Input: dimensioned drawing with shaded views. Units: mm. Origin: part minimum x, y, z. A direction names the side the tool comes from. Give positions to 0.01 mm unless a question says otherwise; leave off trailing zeros. Loops run counter-clockwise (first coordinate to the right, second up) from the corner with the lowest first, then second, coordinate; pieces in that order, holes last. Notation, with made-up numbers: M 26.25,-7.5 L 73.25,-7.5 A15 cw 73.25,17.5 Z; hole C 24,51.5 d11. An arc over 180 degrees is marked long. Use CSV: the item, a comma, the result in double quotes. Start each with the question number.
Q1. Section A-A, the plane z = 10. Output: boundary loops of the cut face in (x, y).
Q2. Reachability of the marked faces 4 and 5 from +Z, -Z, +X, -X, +Y, -Y: full face, straight path, thin tool, end or side. Return the list, or none.
Q3. Section B-B, the plane y = 1.65. Output: boundary loops of the cut face in (x, z).
Q4. Pin query (flat end, axial travel): pin 1 (2.5 mm diameter, centred on x = 10, z = 2.5, fed in from +Y); pin 2 (3 mm diameter, centred on x = 17, z = 15, fed in from +Y); pin 3 (1.5 mm diameter, centred on x = 6, y = 1, fed in from -Z); pin 4 (1 mm diameter, centred on y = 2, z = 5, fed in from +X). Return the tip coordinate at first contact, or that it passes through.
Q5. Section D-D, the plane z = 3.5. Output: boundary loops of the cut face in (x, y), plus the area to 3 significant figures.
Q6. Material intervals for line 1 along X through (y, z) = (0.85, 10); line 2 along X through (y, z) = (4, 10); line 3 along Y through (x, z) = (18.75, 14), sorted ascending.
Q7. Section C-C, the plane x = 10. Output: boundary loops of the cut face in (y, z), plus the area to 3 significant figures.
Q8. Pull-direction query (Z, two-part tool) for the marked faces 1, 2 and 3; classes: released by +Z, released by -Z, zero draft, split by the parting line, or undercut.
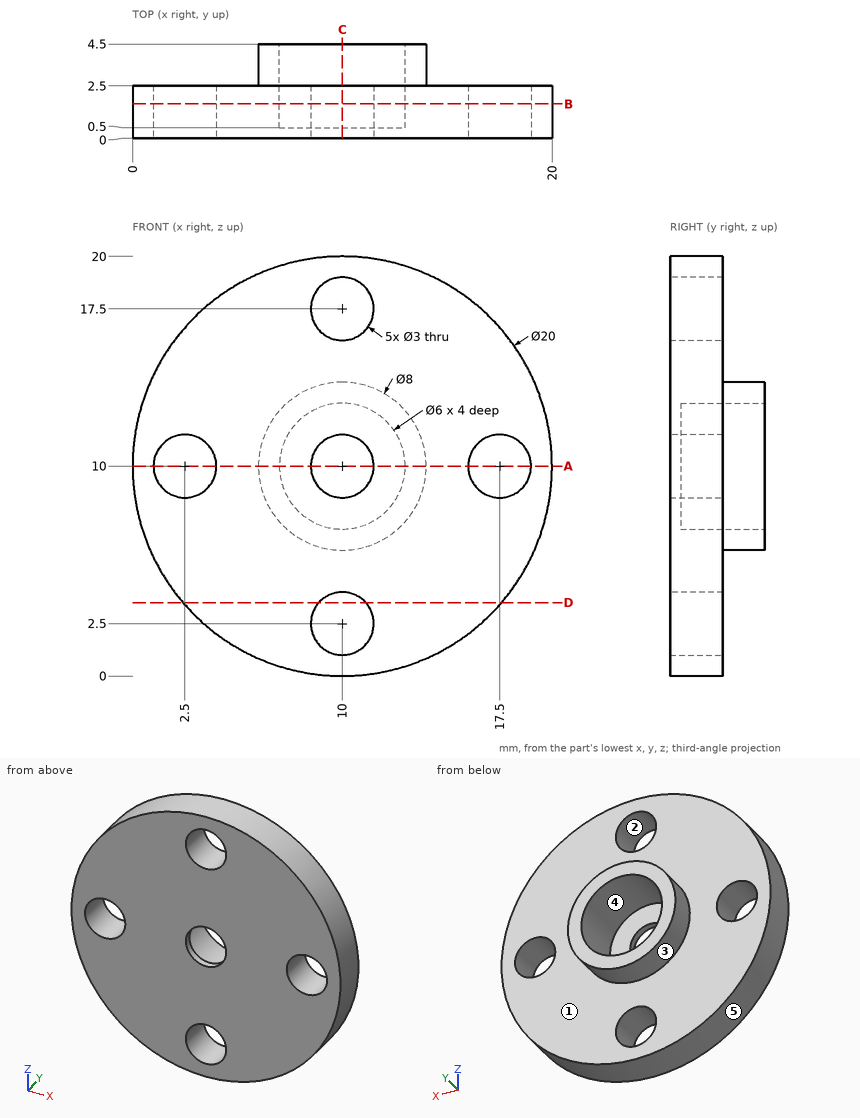
A:
1,outline,"M 0,0 L 1,0 L 1,2.5 L 0,2.5 Z; M 4,0 L 8.5,0 L 8.5,0.5 L 7,0.5 L 7,4.5 L 6,4.5 L 6,2.5 L 4,2.5 Z; M 11.5,0 L 16,0 L 16,2.5 L 14,2.5 L 14,4.5 L 13,4.5 L 13,0.5 L 11.5,0.5 Z; M 19,0 L 20,0 L 20,2.5 L 19,2.5 Z"
2,face 4,"+Y"
2,face 5,"+Y, -Y"
3,outline,"C 10,10 d20; hole C 2.5,10 d3; hole C 10,10 d6; hole C 10,2.5 d3; hole C 10,17.5 d3; hole C 17.5,10 d3"
4,pin 1,"through"
4,pin 2,"y = 2.5"
4,pin 3,"z = 0.54"
4,pin 4,"x = 18.93"
5,outline,"M 2.4,0 L 8.88,0 L 8.88,2.5 L 2.4,2.5 Z; M 11.12,0 L 17.6,0 L 17.6,2.5 L 11.12,2.5 Z"
5,area,"32.4 mm^2"
6,line 1,"0 to 1, 4 to 7, 13 to 16, 19 to 20"
6,line 2,"6 to 7, 13 to 14"
6,line 3,"0 to 2.5"
7,outline,"M 0,0 L 2.5,0 L 2.5,1 L 0,1 Z; M 0,4 L 2.5,4 L 2.5,6 L 4.5,6 L 4.5,7 L 0.5,7 L 0.5,8.5 L 0,8.5 Z; M 0,11.5 L 0.5,11.5 L 0.5,13 L 4.5,13 L 4.5,14 L 2.5,14 L 2.5,16 L 0,16 Z; M 0,19 L 2.5,19 L 2.5,20 L 0,20 Z"
7,area,"25.5 mm^2"
8,face 1,"zero draft"
8,face 2,"undercut"
8,face 3,"split by the parting line"
